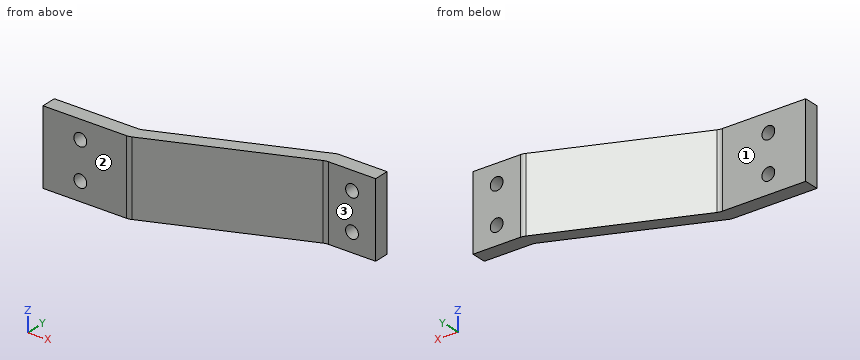
Autodesk Inventor part; units mm, degrees
ref_plane "YZ Plane" through (0, 0, 0) normal (1, 0, 0) x (0, 1, 0)
ref_plane "XZ Plane" through (0, 0, 0) normal (0, 1, 0) x (-1, 0, 0)
ref_plane "XY Plane" through (0, 0, 0) normal (0, 0, 1) x (1, 0, 0)
sketch "Sketch1" plane through (0, 0, 0) normal (0, 0, 1) x (1, 0, 0)
  line L0 (5.715, 0) -> (82.169, 31.75)
  line L1 (82.169, 31.75) -> (107.569, 31.75)
  line L2 (107.569, 31.75) -> (107.569, 24.13)
  line L3 (107.569, 24.13) -> (82.169, 24.13)
  line L4 (82.169, 24.13) -> (5.715, -7.62)
  line L5 (5.715, -7.62) -> (-38.1, -7.62)
  line L6 (-38.1, 0) -> (-38.1, -7.62)
  line L7 (-38.1, 0) -> (5.715, 0)
  point P0 (0, 0)
  dimension "d8" = 7.62
  dimension "d9" = 7.62
  dimension "d13" = 145.669
  dimension "d21" = 38.1
  dimension "d22" = 5.715
  dimension "d23" = 43.815
  dimension "d24" = 76.454
  dimension "d25" = 25.4
  dimension "d26" = 7.62
  dimension "d49" = 31.75
extrude "Extrusion1" add sketch "Sketch1" along normal blind 38.1
fillet "Fillet1" radius 6.35 4 edges at (5.715, -7.62, 19.05) (5.715, 0, 19.05) (82.169, 31.75, 19.05) (82.169, 24.13, 19.05)
sketch "Sketch2" plane through (107.569, 24.13, 0) normal (0, -1, 0) x (1, 0, 0)
  line L0 (-24.1339, 0) -> (-24.1339, 38.1)
  line L1 (-24.1339, 0) -> (0, 0)
  line L2 (0, 0) -> (0, 38.1)
  line L3 (-24.1339, 38.1) -> (0, 38.1)
  line L4 (-12.0669, 38.1) -> (-12.0669, 0) construction
  line L5 (0, 19.05) -> (-24.1339, 19.05) construction
  point P0 (-107.569, 0)
  point P1 (-12.0669, 9.525)
  point P2 (-12.0669, 28.575)
  dimension "d30" = 9.525
  dimension "d31" = 9.525
sketch "Sketch3" plane through (-38.1, -7.62, 0) normal (0, -1, 0) x (1, 0, 0)
  line L0 (0, 38.1) -> (42.5489, 38.1)
  line L1 (0, 0) -> (0, 38.1)
  line L2 (0, 0) -> (42.5489, 0)
  line L3 (19.05, 38.1) -> (19.05, 0)
  point P0 (38.1, 0)
  point P1 (19.05, 28.575)
  point P2 (19.05, 9.525)
  dimension "d32" = 19.05
  dimension "d33" = 9.525
  dimension "d34" = 9.525
hole "Hole1" at (95.5021, 24.13, 28.575) at (95.5021, 24.13, 9.525) direction (0, 1, 0) diameter 6.5278 end through all
hole "Hole2" at (-19.05, -7.62, 28.575) at (-19.05, -7.62, 9.525) direction (0, 1, 0) diameter 6.5278 end through all
properties part number "Y_shaft_support_brace_B" material "Aluminum 6061"
Source: CAD feature listing. Evaluate the final solid. Frame: model axes, mm. Face numbers are marked on the shaded views. A direction names the side the tool comes from. Coordinates: 2 decimals unless noted, no trailing zeros. Loops run counter-clockwise (first coordinate to the right, second up) from the corner with the lowest first, then second, coordinate; pieces in that order, holes last. Notation, with made-up numbers: M -33,-7 L -24,-7 A17 ccw -24,26 Z; hole C -36,-29.5 d7. An arc over 180 degrees is marked long. Use a Markdown table: item, result. Add a question column.
Q1. Section query B-B, the plane z = 9. Return loops of the section in (x, y).
Q2. First-contact query: pin 1 (10.5 mm diameter, centred on x = -19.05, z = 28.575, fed in from +Y); pin 2 (5 mm diameter, centred on x = 43, z = 26.5, fed in from +Y); pin 3 (8 mm diameter, centred on x = 39.5, z = 9.5, fed in from -Y). Flat tips, straight axial feed; report the tip coordinate or a pass-through.
Q3. Material intervals for L1, parallel to Y at x = 98, z = 13; L2, parallel to X at y = 25, z = 7 (3 decimals); L3, parallel to X at y = -5, z = 30.5, sorted ascending.
Q4. Section query A-A, the plane x = -19.05. Return loops of the section in (y, z), and give its area (3 significant figures).
Q5. Section query C-C, the plane z = 18. Return loops of the section in (x, y), and give its area (3 significant figures).
Q6. Access query for the marked faces 1, 2 and 3. Directions: +Z, -Z, +X, -X, +Y, -Y. A direction counts if a zero-diameter tool reaches every point of the face in a straight line with its end or side. Return the directions, or none.
Q7. Section query D-D, the plane z = 29. Return loops of the section in (x, y), and give its area (3 significant figures).
Result:
| question | item | result |
|---|---|---|
| 1 | outline | M -38.1,-7.62 L -22.27,-7.62 L -22.27,0 L -38.1,0 Z; M -15.83,-7.62 L 4.45,-7.62 A6.35 ccw 6.88,-7.13 L 81,23.64 A6.35 cw 83.44,24.13 L 92.28,24.13 L 92.28,31.75 L 83.44,31.75 A6.35 ccw 81,31.26 L 6.88,0.49 A6.35 cw 4.45,0 L -15.83,0 Z; M 98.72,24.13 L 107.57,24.13 L 107.57,31.75 L 98.72,31.75 Z |
| 2 | pin 1 | stops at y = 0 |
| 2 | pin 2 | stops at y = 16.52 |
| 2 | pin 3 | stops at y = 4.75 |
| 3 | L1 | y = 24.13 to 31.75 |
| 3 | L2 | x = 65.915 to 93.434, 97.57 to 107.569 |
| 3 | L3 | x = -38.1 to -21.69, -16.41 to 12.02 |
| 4 | outline | M -7.62,0 L 0,0 L 0,6.26 L -7.62,6.26 Z; M -7.62,12.79 L 0,12.79 L 0,25.31 L -7.62,25.31 Z; M -7.62,31.84 L 0,31.84 L 0,38.1 L -7.62,38.1 Z |
| 4 | area | 191 mm2 |
| 5 | outline | M -38.1,-7.62 L 4.45,-7.62 A6.35 ccw 6.88,-7.13 L 81,23.64 A6.35 cw 83.44,24.13 L 107.57,24.13 L 107.57,31.75 L 83.44,31.75 A6.35 ccw 81,31.26 L 6.88,0.49 A6.35 cw 4.45,0 L -38.1,0 Z |
| 5 | area | 1,110 mm2 |
| 6 | face 1 | +Z, -Z, -X, +Y |
| 6 | face 2 | +Z, -Z, +X, -X, -Y |
| 6 | face 3 | +Z, -Z, +X, -Y |
| 7 | outline | M -38.1,-7.62 L -22.29,-7.62 L -22.29,0 L -38.1,0 Z; M -15.81,-7.62 L 4.45,-7.62 A6.35 ccw 6.88,-7.13 L 81,23.64 A6.35 cw 83.44,24.13 L 92.27,24.13 L 92.27,31.75 L 83.44,31.75 A6.35 ccw 81,31.26 L 6.88,0.49 A6.35 cw 4.45,0 L -15.81,0 Z; M 98.74,24.13 L 107.57,24.13 L 107.57,31.75 L 98.74,31.75 Z |
| 7 | area | 1,010 mm2 |
